Geometry: final body of the model. Coordinates: model frame, mm. Coordinates: 2 decimals unless noted, no trailing zeros. Order: outer loops, then holes, each group sorted by start corner. A loop starts at its lowest first (then second) coordinate and runs counter-clockwise, first axis right, second up. Notation, with made-up numbers: (12, 58.25) -> (25, 58.25) arc R14 ccw to (25, 81.25) -> close; hole circle Ø8 at (-7.5, 73). An arc over 180 degrees is marked (long way). Answer in a Markdown table with one row per item. Add a question column.
1) Section query C-C on y = -3.5. Return the cut outline in (x, z), then the cut area to 3 significant figures.
2) Section query B-B on z = 0.4. Return the cut outline in (x, y), then the cut area to 3 significant figures.
3) Section query D-D on x = 2. Return the cut outline in (y, z), then the cut area to 3 significant figures.
4) Section query A-A on x = -6. Return the cut outline in (y, z), then the cut area to 3 significant figures.
5) Ray query, line 1 (Y direction, x = -4, z = 0.7); line 2 (X direction, y = 37, z = 0.9); line 3 (X direction, y = 14.5, z = 0.85). Return the intervals inside material, ascending. Write a range as from..to.
Autodesk Inventor part; units mm, degrees
ref_plane "YZ Plane" through (0, 0, 0) normal (1, 0, 0) x (0, 1, 0)
ref_plane "XZ Plane" through (0, 0, 0) normal (0, 1, 0) x (-1, 0, 0)
ref_plane "XY Plane" through (0, 0, 0) normal (0, 0, 1) x (1, 0, 0)
sketch "Sketch1" plane through (0, 0, 0) normal (0, 0, 1) x (1, 0, 0)
  circle A0 centre (-4.920941, 38.889745) radius 2.1844
  circle A1 centre (-4.920941, 13.489745) radius 2.1844
  circle A2 centre (-15.45714, 1.56974) radius 2.1844
  circle A3 centre (15.262073, -38.889745) radius 2.1844
  circle A4 centre (15.262073, -38.889745) radius 6.35
  circle A5 centre (-15.45714, 1.56974) radius 6.35
  circle A6 centre (-4.920941, 38.889745) radius 6.35
  line L0 (-21.238079, 4.197144) -> (-11.03537, 40.603294)
  line L1 (1.193489, 40.603294) -> (21.408485, -37.294715)
  line L2 (-20.544521, -2.230399) -> (10.204623, -42.729627)
  point P0 (0, 0)
  dimension "d0" = 12.7
  dimension "d1" = 12.7
  dimension "d2" = 12.7
sketch "Sketch1 outline for Extrusion1" plane through (0, 0, 0) normal (0, 0, 1) x (1, 0, 0)
  line L0 (-20.544521, -2.230399) -> (10.204623, -42.729627)
  arc A0 (-21.238079, 4.197144) -> (-20.544521, -2.230399) centre (-15.45714, 1.56974) ccw
  arc A1 (10.204623, -42.729627) -> (21.408485, -37.294715) centre (15.262073, -38.889745) ccw
  line L1 (-11.03537, 40.603294) -> (-21.238079, 4.197144)
  line L2 (21.408485, -37.294715) -> (1.193489, 40.603294)
  arc A2 (1.193489, 40.603294) -> (-11.03537, 40.603294) centre (-4.920941, 38.889745) ccw
  circle A3 centre (15.262073, -38.889745) radius 2.1844
  circle A4 centre (-15.45714, 1.56974) radius 2.1844
  circle A5 centre (-4.920941, 13.489745) radius 2.1844
  circle A6 centre (-4.920941, 38.889745) radius 2.1844
extrude "Extrusion1" add sketch "Sketch1 outline for Extrusion1" along normal blind 1.5875
properties part number "intakesupport"
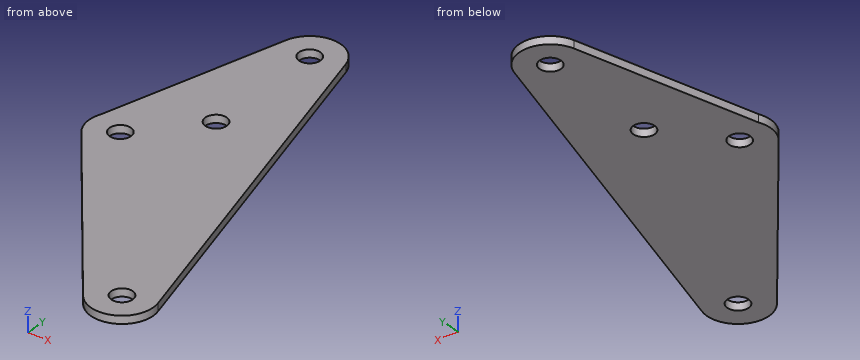
Result:
| question | item | result |
|---|---|---|
| 1 | outline | (-19.58, 0) -> (12.64, 0) -> (12.64, 1.59) -> (-19.58, 1.59) -> close |
| 1 | area | 51.1 mm2 |
| 2 | outline | (-21.24, 4.2) arc R6.35 ccw to (-20.54, -2.23) -> (10.2, -42.73) arc R6.35 ccw to (21.41, -37.29) -> (1.19, 40.6) arc R6.35 ccw to (-11.04, 40.6) -> close; hole circle Ø4.37 at (-15.46, 1.57); hole circle Ø4.37 at (-4.92, 13.49); hole circle Ø4.37 at (-4.92, 38.89); hole circle Ø4.37 at (15.26, -38.89) |
| 2 | area | 1,930 mm2 |
| 3 | outline | (-31.92, 0) -> (37.5, 0) -> (37.5, 1.59) -> (-31.92, 1.59) -> close |
| 3 | area | 110 mm2 |
| 4 | outline | (-21.39, 0) -> (11.59, 0) -> (11.59, 1.59) -> (-21.39, 1.59) -> close; (15.39, 0) -> (36.99, 0) -> (36.99, 1.59) -> (15.39, 1.59) -> close; (40.79, 0) -> (45.15, 0) -> (45.15, 1.59) -> (40.79, 1.59) -> close |
| 4 | area | 93.6 mm2 |
| 5 | line 1 | -24.02..11.51, 15.47..36.91, 40.87..45.17 |
| 5 | line 2 | -12.05..-6.02, -3.83..2.13 |
| 5 | line 3 | -18.35..-6.86, -2.98..7.97 |
